Model file for the job. Use its own axes, mm. Coordinates: 2 decimals unless noted, no trailing zeros. Order: outer loops, then holes, each group sorted by start corner. A loop starts at its lowest first (then second) coordinate and runs counter-clockwise, first axis right, second up. Notation, with made-up numbers: (75.25, 30) -> (116.25, 30) arc R29 cw to (116.25, 55) -> close; hole circle Ø8 at (6.25, 9). An arc over 180 degrees is marked (long way). Return JSON: item names as keys, results as strings. Group by question number.
1) Probe line 1 (Y direction, x = 0, z = 11.5); line 2 (Y direction, x = 0, z = 8.5); line 3 (Z direction, x = -2.5, y = 7) (3 decimals). List the from-to ranges inside material, lowest first.
2) Pull direction X, two halves, no side cores. Call faces 1 (the flat face through (7, 0, 9.525)), 2 (the cylindrical face through (0.84, 6.41, 4.7)), 3 (the cylindrical face through (0.55, 4.18, 7.83)): +X half, -X half, draft (parallel to the pull), parting line (faces both ways), or undercut.
3) Cut at D-D (z = 13.75). Write the cut outline in (x, y) (1 decimal).
4) Cut at C-C (z = 5.25). Write the cut outline in (x, y), and give its area (3 significant figures).
5) Flat gauge pins, fed straight in: pin 1 (3 mm diameter, centred on y = 0.5, z = 3, fed in from +X); pin 2 (5 mm diameter, centred on y = 6, z = 12.5, fed in from +X); pin 3 (4 mm diameter, centred on y = 5, z = 7, fed in from -X). Where does each tip first touch, or does it go through?
from build123d import *

# Parameters (mm, degrees)
SKETCH1_R                   = 7.9375
BOSS_EXTRUDE1_DEPTH         = 15.875
CHAMFER1_SIZE               = 0.254
SKETCH2_OUTSIDE_W           = 23.376
SKETCH2_OUTSIDE_H           = 23.376
SKETCH2_OUTSIDE_R           = 6.4643
CUT_EXTRUDE1_DEPTH          = 9.525
TAP_DRILL_FOR_3_8_24_TAP1_D = 8.4328


with BuildPart() as part:
    # Sketch1 → Boss-Extrude1 (new body)
    with BuildSketch(Plane.XY):
        Circle(SKETCH1_R)
    extrude(amount=BOSS_EXTRUDE1_DEPTH)

    # Chamfer1
    chamfer1_edges = [part.edges().sort_by_distance(p)[0] for p in [
        (-7.9375, 0, 15.875),
    ]]
    chamfer(chamfer1_edges, length=CHAMFER1_SIZE)

    # Sketch2 outside → Cut-Extrude1 (cut)
    with BuildSketch(Plane(origin=(0, 0, 0), x_dir=(-1, 0, 0), z_dir=(0, 0, -1))):
        Rectangle(SKETCH2_OUTSIDE_W, SKETCH2_OUTSIDE_H)
        Circle(SKETCH2_OUTSIDE_R, mode=Mode.SUBTRACT)
    extrude(amount=-CUT_EXTRUDE1_DEPTH, mode=Mode.SUBTRACT)

    # Tap Drill for 3/8-24 Tap1 (through all)
    with Locations(Plane.XY.offset(15.875)):
        with Locations((0, 0)):
            Hole(TAP_DRILL_FOR_3_8_24_TAP1_D / 2)


solid = part.part
Answers below:
{
 "1": {"line 1": "y = -7.94 to -4.22, 4.22 to 7.94", "line 2": "y = -6.46 to -4.22, 4.22 to 6.46", "line 3": "z = 9.525 to 15.875"},
 "2": {"face 1": "draft", "face 2": "parting line", "face 3": "undercut"},
 "3": {"outline": "circle Ø15.9 at (0, 0); hole circle Ø8.4 at (0, 0)"},
 "4": {"outline": "circle Ø12.93 at (0, 0); hole circle Ø8.43 at (0, 0)", "area": "75.4 mm^2"},
 "5": {"pin 1": "stops at x = 6.46", "pin 2": "stops at x = 7.12", "pin 3": "stops at x = -5.73"}
}
